from build123d import *

# Parameters (mm, degrees)
F0_R     = 24.6407152677
F1_DEPTH = 51.562
F2_SIZE  = 5.08
F3_DEPTH = 25.4
F4_R     = 22.86


with BuildPart() as f1:
    # F0 (on Top) → F1 (new body)
    with BuildSketch(Plane.XY):
        Circle(F0_R)
    extrude(amount=F1_DEPTH)

    # F2
    f2_edges = [f1.edges().sort_by_distance(p)[0] for p in [
        (-24.640715, 0, 0),
    ]]
    chamfer(f2_edges, length=F2_SIZE)

    # F3 (add): a face of the model
    f3_faces = [f1.faces().sort_by_distance(p)[0] for p in [
        (0, 0, 51.562),
    ]]
    extrude(f3_faces, amount=F3_DEPTH)

    # F4
    f4_edges = [f1.edges().sort_by_distance(p)[0] for p in [
        (-24.640715, 0, 76.962),
    ]]
    fillet(f4_edges, radius=F4_R)


solid = f1.part
Could you check a few things on this model? Use its own coordinates, in mm. Round coordinates to 2 decimals unless told otherwise and drop trailing zeros. Order: outer loops, then holes, each group sorted by start corner. A loop starts at its lowest first (then second) coordinate and runs counter-clockwise, first axis right, second up.
Q1. I'm going to push flat-ended pins straight in: P1, Ø8, axis at x = 17, z = 47.5, coming from the -Y side; P2, Ø6, axis at x = 7.5, y = -6, coming from the +Z side; P3, Ø4, axis at x = -4, z = 50.5, coming from the +Y side. Where does each tip first touch, or does it pass through?
Geometry says:
P1: stops at y = -20.93
P2: stops at z = 76.45
P3: stops at y = 24.56
Q2. Please list where these lines run through material, in increasing order: probe 1 along Z at (x, y) = (-5, -7); probe 2 along Z at (x, y) = (-2.5, -7); probe 3 along Y at (x, z) = (0, 14.5).
Geometry says:
probe 1: z = 0 to 75.92
probe 2: z = 0 to 76.25
probe 3: y = -24.64 to 24.64
Q3. Imagine slicing it at A-A, the plane z = 41. List the corners of the cut face in (x, y) for me, then the cut area to 3 significant figures.
Geometry says:
outline: circle Ø49.28 at (0, 0)
area: 1,910 mm2
